Model file for the job. Use its own axes, mm. Face numbers are marked on the shaded views. A direction names the side the tool comes from. Round coordinates to 2 decimals unless told otherwise and drop trailing zeros. Order: outer loops, then holes, each group sorted by start corner. A loop starts at its lowest first (then second) coordinate and runs counter-clockwise, first axis right, second up. Notation, with made-up numbers: M 81.25,17 L 104.25,17 A18 cw 104.25,40 Z; hole C 63,-15 d3. An arc over 180 degrees is marked long. Return JSON: item names as keys, results as strings. Group by question number.
Item 1: Pull direction Y, two halves, no side cores. Call the marked faces 4, 5 and 6: pulls with the +Y half, pulls with the -Y half, needs draft (parallel to the pull), parting line crosses it, or undercut.
Item 2: Slice it at B-B on x = -5.5. Write the cut outline in (y, z).
Item 3: Slice it at A-A on y = 0. Write the cut outline in (x, z).
Item 4: Which spindle directions (+Z, -Z, +X, -X, +Y, -Y) get a long thin tool onto all of the face, cutting with end or side? Do the marked faces 1, 2 and 3. Say none if no direction does.
Item 5: Slice it at D-D on z = 100. Write the cut outline in (x, y).
Item 6: Slice it at C-C on z = 197.5. Write the cut outline in (x, y).
Item 7: Pin check, flat tips, straight feed: pin 1 Ø8 at (y, z) = (0, 179.5) entering from +X; pin 2 Ø7.5 at (x, y) = (-5.5, 65) entering from +Z; pin 3 Ø12 at (x, z) = (117, 35) entering from +Y. Stop position of each tip, or through.
Item 8: Probe line 1 along Y through (x, z) = (74.5, 137); line 2 along Z through (x, y) = (97.5, 14); line 3 along X through (y, z) = (37.5, 176). List the from-to ranges inside material, lowest first.
from build123d import *

# Parameters (mm, degrees)
F0_W     = 310
F0_H     = 136.5
F1_DEPTH = 160.5
F2_R     = 52
F2_R_2   = 50
F3_DEPTH = 60.3
F4_R     = 76
F4_R_2   = 52
F4_R_3   = 50
F5_DEPTH = 21.3
F7_D     = 8.4
F7_DEPTH = 24
F7_TIP   = 2.5236145999


with BuildPart() as f1:
    # F0 (on Top) → F1 (new body)
    with BuildSketch(Plane.XY):
        Rectangle(F0_W, F0_H)
    extrude(amount=F1_DEPTH)

    # F2 (on face) → F3 (join)
    with BuildSketch(Plane.XY.offset(160.5)):
        with Locations((-5.5, 0)):
            Circle(F2_R)
        with Locations((-5.5, 0)):
            Circle(F2_R_2, mode=Mode.SUBTRACT)
    extrude(amount=F3_DEPTH)

    # F4 (on face) → F5 (join)
    with BuildSketch(Plane.XY.offset(220.8)):
        with Locations((-5.5, 0)):
            Circle(F4_R)
        with Locations((-5.5, 0)):
            Circle(F4_R_2, mode=Mode.SUBTRACT)
        with Locations((-5.5, 0)):
            Circle(F4_R_2)
        with Locations((-5.5, 0)):
            Circle(F4_R_3, mode=Mode.SUBTRACT)
    extrude(amount=F5_DEPTH)

    # F7
    with Locations(Plane.XY.offset(242.1)):
        with Locations((-5.5, 65), (19.3744231037, 60.0521696132), (40.4619407771, 45.9619407771), (54.5521696132, 24.8744231037), (59.5, 0), (54.5521696132, -24.8744231037), (40.4619407771, -45.9619407771), (19.3744231037, -60.0521696132), (-5.5, -65), (-30.3744231037, -60.0521696132), (-51.4619407771, -45.9619407771), (-65.5521696132, -24.8744231037), (-70.5, 0), (-65.5521696132, 24.8744231037), (-51.4619407771, 45.9619407771), (-30.3744231037, 60.0521696132)):
            Hole(F7_D / 2, depth=F7_DEPTH)
            with Locations((0, 0, -(F7_DEPTH + F7_TIP / 2))):  # 118° drill point
                Cone(0, F7_D / 2, F7_TIP, mode=Mode.SUBTRACT)


solid = f1.part
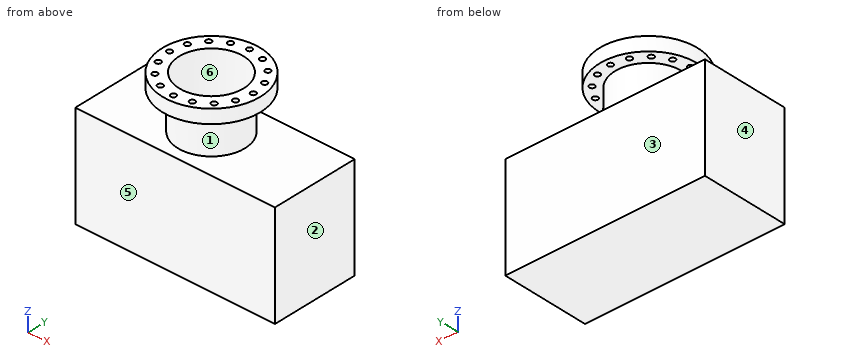
Output values:
{
 "1": {"face 4": "needs draft", "face 5": "pulls with the -Y half", "face 6": "undercut"},
 "2": {"outline": "M -76,220.8 L -69.2,220.8 L -69.2,242.1 L -76,242.1 Z; M -68.25,0 L 68.25,0 L 68.25,160.5 L 52,160.5 L 52,220.8 L 60.8,220.8 L 60.8,242.1 L 50,242.1 L 50,160.5 L -50,160.5 L -50,242.1 L -60.8,242.1 L -60.8,220.8 L -52,220.8 L -52,160.5 L -68.25,160.5 Z; M 69.2,220.8 L 76,220.8 L 76,242.1 L 69.2,242.1 Z"},
 "3": {"outline": "M -155,0 L 155,0 L 155,160.5 L 46.5,160.5 L 46.5,220.8 L 55.3,220.8 L 55.3,242.1 L 44.5,242.1 L 44.5,160.5 L -55.5,160.5 L -55.5,242.1 L -66.3,242.1 L -66.3,220.8 L -57.5,220.8 L -57.5,160.5 L -155,160.5 Z; M -81.5,220.8 L -74.7,220.8 L -74.7,242.1 L -81.5,242.1 Z; M 63.7,220.8 L 70.5,220.8 L 70.5,242.1 L 63.7,242.1 Z"},
 "4": {"face 1": "none", "face 2": "+Z, -Z, +X, +Y, -Y", "face 3": "-Z, +X, -X, +Y"},
 "5": {"outline": "M -155,-68.25 L 155,-68.25 L 155,68.25 L -155,68.25 Z"},
 "6": {"outline": "C -5.5,0 d104; hole C -5.5,0 d100"},
 "7": {"pin 1": "x = 46.5", "pin 2": "z = 160.5", "pin 3": "y = 68.25"},
 "8": {"line 1": "-68.25 to 68.25", "line 2": "0 to 160.5", "line 3": "-41.52 to -38.57, 27.57 to 30.52"}
}
